Here's how the part is built. I have some questions about the finished solid (model axes, mm). Coordinates: 2 decimals unless noted, no trailing zeros. Order: outer loops, then holes, each group sorted by start corner. A loop starts at its lowest first (then second) coordinate and runs counter-clockwise, first axis right, second up. Notation, with made-up numbers: (84, -26.75) - (106, -26.75) arc R30 cw to (106, -4.75) - close; hole circle Ø7 at (23.25, 20.25). An arc over 180 degrees is marked (long way). Answer in a Markdown table with one row per item. Add a question column.
Item 1: I want a section at D-D (x = -25.7). Count the separate pieces of the cut face and the enclosed holes in it, plus the area to 3 significant figures.
Item 2: I want a section at B-B (y = -32). Please give me the cut outline in (x, z) (3 decimals).
Item 3: Will this pin go through, and if not, where does the flat tip stop? pin 1 Ø1.5 at (x, z) = (-22.5, 12.5) entering from +Y.
Item 4: If I drill on line 1 along Z through (x, y) = (-24.3, -33); line 2 along Z through (x, y) = (-22.45, -34); line 3 along Y through (x, z) = (-25.35, 16.5), over which ranges is the centre line in solid material (lowest first)? Write a range as from..to.
Item 5: I want a section at C-C (y = 78). Please give me the cut outline in (x, z), plus the area to 3 significant figures.
Item 6: I want a section at A-A (z = -38.5). Please give me the cut outline in (x, y).
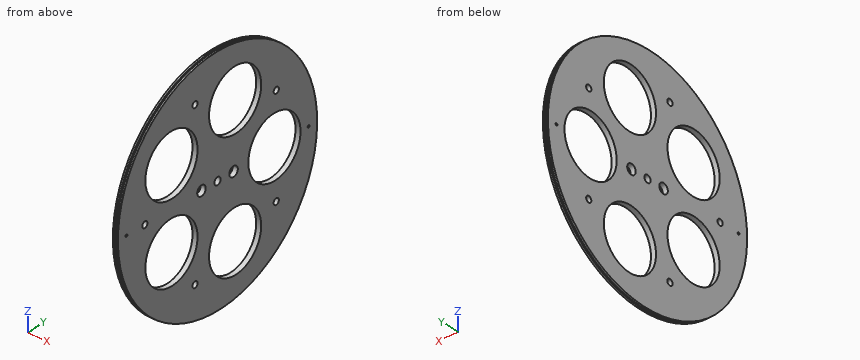
```python
from build123d import *

# Parameters (mm, degrees)
SKETCH_22_R         = 3.3
SKETCH_22_R_2       = 4.5
SKETCH_22_R_3       = 1
SKETCH_22_R_4       = 27.5
SKETCH_22_R_5       = 2.75
CUT_EXTRUDE_1_DEPTH = 10


with BuildPart() as part:
    # 草图1 → 旋转1 (revolve)
    with BuildSketch(Plane.XY, mode=Mode.PRIVATE) as revolve_1_sk:
        Polygon((-21.9, 11), (-21.9, 25), (-21.9, 105), (-23, 105), (-23.6, 105), (-23.6, 95), (-24.2, 95), (-24.8, 95), (-24.8, 105), (-25, 105), (-26.5, 105), (-26.5, 98.307417596), (-26.5, 11), (-26.5, 0), (-21.9, 0), align=None)
    revolve(revolve_1_sk.sketch.rotate(Axis((-21, 0, 0), (1, 0, 0)), 90), axis=Axis((-21, 0, 0), (1, 0, 0)))

    # 草图22 → 切除-拉伸1 (cut)
    with BuildSketch(Plane(origin=(-21.9, 0, 0), x_dir=(0, 0, -1), z_dir=(1, 0, 0))):
        Circle(SKETCH_22_R)
        with Locations((0, 16.9)):
            Circle(SKETCH_22_R_2)
        with Locations((0, 96)):
            Circle(SKETCH_22_R_3)
        with Locations((0, 60)):
            Circle(SKETCH_22_R_4)
        with Locations((0, -16.9)):
            Circle(SKETCH_22_R_2)
        with Locations((57.063390978, 18.541019662)):
            Circle(SKETCH_22_R_4)
        with Locations((72.794835514, -23.652475842)):
            Circle(SKETCH_22_R_5)
        with Locations((35.267115138, -48.541019662)):
            Circle(SKETCH_22_R_4)
        with Locations((-35.267115138, -48.541019662)):
            Circle(SKETCH_22_R_4)
        with Locations((-57.063390978, 18.541019662)):
            Circle(SKETCH_22_R_4)
        with Locations((0, -96)):
            Circle(SKETCH_22_R_3)
        with Locations((0, -76.541019662)):
            Circle(SKETCH_22_R_5)
        with Locations((-72.794835514, -23.652475842)):
            Circle(SKETCH_22_R_5)
        with Locations((-44.989682553, 61.922985674)):
            Circle(SKETCH_22_R_5)
        with Locations((44.989682553, 61.922985674)):
            Circle(SKETCH_22_R_5)
    extrude(amount=-CUT_EXTRUDE_1_DEPTH, mode=Mode.SUBTRACT)


solid = part.part
```
Values follow:
| question | item | result |
|---|---|---|
| 1 | separate pieces | 1 |
| 1 | enclosed holes | 15 |
| 1 | area | 22,500 mm^2 |
| 2 | outline | (-26.5, -100.005) - (-24.8, -100.005) - (-24.8, -89.448) - (-23.6, -89.448) - (-23.6, -100.005) - (-21.9, -100.005) - (-21.9, -57.236) - (-26.5, -57.236) - close; (-26.5, -13.298) - (-21.9, -13.298) - (-21.9, 13.298) - (-26.5, 13.298) - close; (-26.5, 57.236) - (-21.9, 57.236) - (-21.9, 100.005) - (-23.6, 100.005) - (-23.6, 89.448) - (-24.8, 89.448) - (-24.8, 100.005) - (-26.5, 100.005) - close |
| 3 | pin 1 | stops at y = 104.34 |
| 4 | line 1 | z = -89.08..-57.95, -12.58..12.58, 57.95..89.08 |
| 4 | line 2 | z = -99.34..-58.61, -11.93..11.93, 58.61..99.34 |
| 4 | line 3 | y = -103.7..-68.64, -28.44..38, 82..103.7 |
| 5 | outline | (-26.5, -70.29) - (-24.8, -70.29) - (-24.8, -54.23) - (-23.6, -54.23) - (-23.6, -70.29) - (-21.9, -70.29) - (-21.9, -20.79) - (-26.5, -20.79) - close; (-26.5, 20.79) - (-21.9, 20.79) - (-21.9, 70.29) - (-23.6, 70.29) - (-23.6, 54.23) - (-24.8, 54.23) - (-24.8, 70.29) - (-26.5, 70.29) - close |
| 5 | area | 417 mm^2 |
| 6 | outline | (-26.5, -97.69) - (-24.8, -97.69) - (-24.8, -86.85) - (-23.6, -86.85) - (-23.6, -97.69) - (-21.9, -97.69) - (-21.9, -75.85) - (-26.5, -75.85) - close; (-26.5, -21.23) - (-21.9, -21.23) - (-21.9, -1.75) - (-26.5, -1.75) - close; (-26.5, 38.83) - (-21.9, 38.83) - (-21.9, 97.69) - (-23.6, 97.69) - (-23.6, 86.85) - (-24.8, 86.85) - (-24.8, 97.69) - (-26.5, 97.69) - close |
